Read the model definition and answer for the solid it produces. Units are mm, in the model's axes. A direction names the side the tool comes from. Round coordinates to 2 decimals unless told otherwise and drop trailing zeros. Order: outer loops, then holes, each group sorted by start corner. A loop starts at its lowest first (then second) coordinate and runs counter-clockwise, first axis right, second up.
Autodesk Fusion 360 part; units mm, degrees
sketch "Sketch2" plane through (0, 0, 0) normal (0, 1, 0) x (1, 0, 0)
  line L0 (20, -1.5) -> (-20, -1.5)
  line L1 (-20, -1.5) -> (-20, 1.5)
  line L2 (-20, 1.5) -> (20, 1.5)
  line L3 (20, 1.5) -> (20, -1.5)
  line L4 (20, -1.5) -> (-20, 1.5) construction
  line L5 (-20, -1.5) -> (20, 1.5) construction
  line L6 (0, -1.5) -> (0, 1.5) construction
  arc A0 (-20, 1.5) -> (0, 1.5) centre (-10, 18.8205) ccw
  arc A1 (0, 1.5) -> (20, 1.5) centre (10, 18.8205) ccw
  line L7 (-20, 1.5) -> (-22.5, 1.5)
  line L8 (-22.5, 1.5) -> (-22.5, -1.5)
  line L9 (-22.5, -1.5) -> (-20, -1.5)
  line L10 (-20, -1.5) -> (-20, 1.5)
  line L11 (20, 1.5) -> (22.5, 1.5)
  line L12 (22.5, 1.5) -> (22.5, -1.5)
  line L13 (22.5, -1.5) -> (20, -1.5)
  line L14 (20, -1.5) -> (20, 1.5)
  dimension "d3" = 3
  dimension "d4" = 40
  dimension "d5" = 20
  dimension "d6" = 20
  dimension "d11" = 2.5
  dimension "d12" = 2.5
extrude "Extrude1" add sketch "Sketch2" along normal blind 19.5 contours L0 L1 L3 A0 A1 L10 L14 | L3 L11 L12 L13 L14 | L1 L7 L8 L9 L10
extrude "Extrude2" add 1 faces at (7.5, 13, 1.5) along direction (0, 0, 1) blind 0.5
sketch "Sketch3" plane through (0, 0, 2) normal (0, 0, 1) x (-1, 0, 0)
  line L0 (22.5, 0) -> (-22.5, 0)
  line L1 (-22.5, 0) -> (-22.5, -19.5)
  line L2 (-22.5, -19.5) -> (22.5, -19.5)
  line L3 (22.5, -19.5) -> (22.5, 0)
  line L4 (22.5, -9.75) -> (-22.5, -9.75) construction
  line L5 (0, -19.5) -> (0, 0) construction
  circle A0 centre (19.5, -9.75) radius 1.5
  dimension "d13" = 3
  dimension "d14" = 3
extrude "Extrude3" add sketch "Sketch3" along normal blind 2 contours A0
sketch "Sketch4" plane through (0, 0, 4) normal (0, 0, 1) x (-1, 0, 0)
  circle A0 centre (19.5, -9.75) radius 1.5
  circle A1 centre (19.5, -9.75) radius 2.5
  dimension "d17" = 5
extrude "Extrude4" add sketch "Sketch4" along normal blind 1.5 contours A0 | A1
ref_plane "WorkPlane1" through (0, 9.75, 0.25) normal (-1, 0, 0) x (0, 0, 1)
mirror "Mirror1" about plane through (0, 9.75, 0.25) normal (-1, 0, 0) of "Extrude3", "Extrude4"
equation "d7 = 16.5 mm + 3 mm"
Q1. For faces 5 (the face through (10.15, 9.61, 1.18)), 6 (the face through (18, 9.7, 3)), 7 (the face through (-17.516, 8.229, 4.74)), determine the directions among +Z, -Z, +X, -X, +Y, -Y from which every point of the face is accessible in a straight line to the end or side of a thin tool.
Outcome:
face 5: -Z, +Y, -Y
face 6: none
face 7: +Z
Q2. A cutting plane is placed at D-D, the plane x = 19.5. Give the vertices of the cut face in (y, z), plus the area to 3 significant figures.
Outcome:
outline: (0, -1.22) - (19.5, -1.22) - (19.5, 2) - (11.25, 2) - (11.25, 4) - (12.25, 4) - (12.25, 5.5) - (7.25, 5.5) - (7.25, 4) - (8.25, 4) - (8.25, 2) - (0, 2) - close
area: 76.3 mm2
Q3. For a pull along X with two mould halves and no side action, classify faces 1 (the face through (-21, 10, -1.5)), 2 (the face through (-18, 9.8, 3)), 3 (the face through (22.5, 10, 0)), 4 (the face through (18, 11, 4)) as released by +X, released by -X, zero draft, split by the parting line, or undercut.
Outcome:
face 1: zero draft
face 2: undercut
face 3: released by +X
face 4: undercut
Q4. A cutting plane is placed at A-A, the plane y = 9.75. Give the vertices of the cut face in (x, z), plus the area to 3 significant figures.
Outcome:
outline: (-22.5, -1.5) - (-20, -1.5) arc R20 cw to (0, -1.5) arc R20 cw to (20, -1.5) - (22.5, -1.5) - (22.5, 2) - (21, 2) - (21, 4) - (22, 4) - (22, 5.5) - (17, 5.5) - (17, 4) - (18, 4) - (18, 2) - (-18, 2) - (-18, 4) - (-17, 4) - (-17, 5.5) - (-22, 5.5) - (-22, 4) - (-21, 4) - (-21, 2) - (-22.5, 2) - close
area: 112 mm2
Q5. A cutting plane is placed at C-C, the plane y = 15. Give the vertices of the cut face in (x, z), plus the area to 3 significant figures.
Outcome:
outline: (-22.5, -1.5) - (-20, -1.5) arc R20 cw to (0, -1.5) arc R20 cw to (20, -1.5) - (22.5, -1.5) - (22.5, 2) - (-22.5, 2) - close
area: 85.0 mm2
Q6. Flat-ended cylindrical pins translate along their axes: pin 1 (3 mm diameter, centred on x = 17, y = 11.5, fed in from -Z); pin 2 (1 mm diameter, centred on x = -11, z = 3, fed in from +Y); pin 3 (2 mm diameter, centred on x = 8.5, y = 5, fed in from +Z); pin 4 (3 mm diameter, centred on x = -12, y = 13.5, fed in from -Z). Find the tip coordinate at first contact, or state that the pin passes through.
Outcome:
pin 1: stops at z = -0.72
pin 2: passes through
pin 3: stops at z = 2
pin 4: stops at z = 0.87
Q7. A cutting plane is placed at B-B, the plane x = -19. Give the vertices of the cut face in (y, z), plus the area to 3 significant figures.
Outcome:
outline: (0, -0.96) - (19.5, -0.96) - (19.5, 2) - (11.16, 2) - (11.16, 4) - (12.2, 4) - (12.2, 5.5) - (7.3, 5.5) - (7.3, 4) - (8.34, 4) - (8.34, 2) - (0, 2) - close
area: 70.7 mm2
Q8. Straight lines are drawn through the part: probe 1 along X at (y, z) = (8.5, -0.75); probe 2 along Y at (x, z) = (17.5, 4.75); probe 3 along Z at (x, y) = (10, 18.5). For each, find the intervals that lie inside material, in ascending order.
Outcome:
probe 1: x = -22.5 to -18.57, -1.43 to 1.43, 18.57 to 22.5
probe 2: y = 8.25 to 11.25
probe 3: z = 1.18 to 2
